Verification items for the finished model (mm, model axes). Coordinates: 2 decimals unless noted, no trailing zeros. Order: outer loops, then holes, each group sorted by start corner. A loop starts at its lowest first (then second) coordinate and runs counter-clockwise, first axis right, second up. Notation, with made-up numbers: (-13, 49.25) -> (32, 49.25) arc R18 cw to (32, 75.25) -> close; hole circle Ø2 at (-13, 53). An arc over 180 degrees is marked (long way). Answer as CSV lines item,"result".
```python
from build123d import *

# Parameters (mm, degrees)
SKETCH1_R           = 2.5
BOSS_EXTRUDE1_DEPTH = 2
CHAMFER1_SIZE       = 0.5


with BuildPart() as part:
    # Sketch1 → Boss-Extrude1 (new body)
    with BuildSketch(Plane.XY):
        with BuildLine():
            ThreePointArc((17.928932188, -7.071067812), (35, 0), (17.928932188, 7.071067812))
            ThreePointArc((17.928932188, 7.071067812), (12.5, 4.82233047), (7.071067812, 7.071067812))
            ThreePointArc((7.071067812, 7.071067812), (-10, 0), (7.071067812, -7.071067812))
            ThreePointArc((7.071067812, -7.071067812), (12.5, -4.82233047), (17.928932188, -7.071067812))
        make_face()
        with Locations((25, 0)):
            Circle(SKETCH1_R, mode=Mode.SUBTRACT)
        Circle(SKETCH1_R, mode=Mode.SUBTRACT)
    extrude(amount=BOSS_EXTRUDE1_DEPTH)

    # Chamfer1
    chamfer1_edges = [part.edges().sort_by_distance(p)[0] for p in [
        (12.5, -4.82233047, 2),
        (-10, 0, 2),
        (12.5, 4.82233047, 2),
        (-10, 0, 0),
        (12.5, -4.82233047, 0),
        (35, 0, 0),
        (12.5, 4.82233047, 0),
        (35, 0, 2),
    ]]
    chamfer(chamfer1_edges, length=CHAMFER1_SIZE)


solid = part.part
```
Item 1: Section check C-C, the plane z = 0.8. Record the boundary of the cut face in (x, y), plus the area to 3 significant figures.
Answer list:
outline,"(7.07, -7.07) arc R7.68 cw to (17.93, -7.07) arc R10 ccw (long way) to (17.93, 7.07) arc R7.68 cw to (7.07, 7.07) arc R10 ccw (long way) to start; hole circle Ø5 at (0, 0); hole circle Ø5 at (25, 0)"
area,"652 mm2"
Item 2: Thickness scan on line 1 (Y direction, x = 25, z = 1.3); line 2 (X direction, y = -1.75, z = 0.5); line 3 (X direction, y = 5.5, z = 0.9). Record the ranges inside material, lowest first.
Answer list:
line 1,"-10 to -2.5, 2.5 to 10"
line 2,"-9.85 to -1.79, 1.79 to 23.21, 26.79 to 34.85"
line 3,"-8.35 to 9.35, 15.65 to 33.35"
Item 3: Release check for a two-part mould opening along X. For faces 1 (the flat face through (12, 0, 0)), 2 (the cylindrical face through (22.5, 0.1, 1)) record: +X half, -X half, draft (parallel to the pull), parting line (faces both ways), or undercut.
Answer list:
face 1,"draft"
face 2,"undercut"
Item 4: Section check B-B, the plane x = 0. Record the boundary of the cut face in (y, z), plus the area to 3 significant figures.
Answer list:
outline,"(-10, 0.5) -> (-9.5, 0) -> (-2.5, 0) -> (-2.5, 2) -> (-9.5, 2) -> (-10, 1.5) -> close; (2.5, 0) -> (9.5, 0) -> (10, 0.5) -> (10, 1.5) -> (9.5, 2) -> (2.5, 2) -> close"
area,"29.5 mm2"
Item 5: Section check A-A, the plane y = 0. Record the boundary of the cut face in (x, z).
Answer list:
outline,"(-10, 0.5) -> (-9.5, 0) -> (-2.5, 0) -> (-2.5, 2) -> (-9.5, 2) -> (-10, 1.5) -> close; (2.5, 0) -> (22.5, 0) -> (22.5, 2) -> (2.5, 2) -> close; (27.5, 0) -> (34.5, 0) -> (35, 0.5) -> (35, 1.5) -> (34.5, 2) -> (27.5, 2) -> close"
